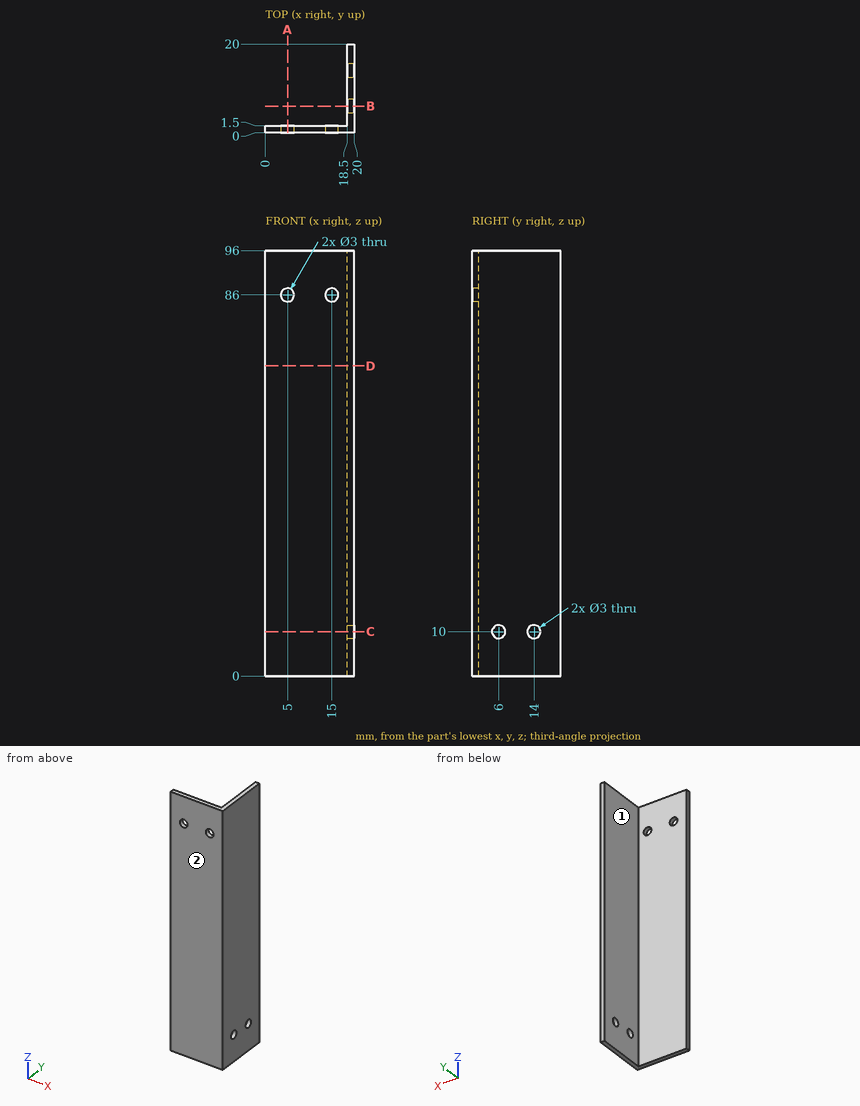
Job drawing, mm, ordinate dimensions from the low corner. One solid piece. A direction names the side the tool comes from. Coordinates: 2 decimals unless noted, no trailing zeros. Order: outer loops, then holes, each group sorted by start corner. A loop starts at its lowest first (then second) coordinate and runs counter-clockwise, first axis right, second up. Notation, with made-up numbers: (56.25, 4) -> (91.25, 4) arc R35 cw to (91.25, 42) -> close; hole circle Ø6 at (12.5, 74.5). An arc over 180 degrees is marked (long way). Put each result on its own line as item: value. Start each with the question number.
(1) Pin check, flat tips, straight feed: pin 1 Ø4 at (x, z) = (5, 86) entering from +Y; pin 2 Ø5.5 at (y, z) = (14, 72) entering from -X; pin 3 Ø2.5 at (y, z) = (6, 10) entering from +X. Stop position of each tip, or through.
(2) Probe line 1 along X through (y, z) = (0.85, 86); line 2 along Z through (x, y) = (5, 1.25); line 3 along X through (y, z) = (5, 51.5). List the from-to ranges inside material, lowest first. Write a range as [from, to].
(3) Band-saw the part on A-A (x = 5). Give the cut face in (y, z).
(4) Band-saw the part on B-B (y = 6). Give the cut face in (x, z).
(5) Band-saw the part on D-D (z = 70). Give the cut face in (x, y).
(6) Band-saw the part on C-C (z = 10). Give the cut face in (x, y).
(7) Which spindle directions (+Z, -Z, +X, -X, +Y, -Y) get a long thin tool onto all of the face, cutting with end or side? Do the marked faces 1 and 2. Say none if no direction does.
Determined:
1. pin 1: stops at y = 1.5
1. pin 2: stops at x = 18.5
1. pin 3: passes through
2. line 1: x = [0, 3.5], [6.5, 13.5], [16.5, 20]
2. line 2: z = [0, 84.5], [87.5, 96]
2. line 3: x = [18.5, 20]
3. outline: (0, 0) -> (1.5, 0) -> (1.5, 84.5) -> (0, 84.5) -> close; (0, 87.5) -> (1.5, 87.5) -> (1.5, 96) -> (0, 96) -> close
4. outline: (18.5, 0) -> (20, 0) -> (20, 8.5) -> (18.5, 8.5) -> close; (18.5, 11.5) -> (20, 11.5) -> (20, 96) -> (18.5, 96) -> close
5. outline: (0, 0) -> (20, 0) -> (20, 20) -> (18.5, 20) -> (18.5, 1.5) -> (0, 1.5) -> close
6. outline: (0, 0) -> (20, 0) -> (20, 4.5) -> (18.5, 4.5) -> (18.5, 1.5) -> (0, 1.5) -> close; (18.5, 7.5) -> (20, 7.5) -> (20, 12.5) -> (18.5, 12.5) -> close; (18.5, 15.5) -> (20, 15.5) -> (20, 20) -> (18.5, 20) -> close
7. face 1: +Z, -Z, -X, +Y
7. face 2: +Z, -Z, +X, -X, -Y
